from build123d import *

# Parameters (mm, degrees)
SKETCH1_R           = 2.7
BOSS_EXTRUDE1_DEPTH = 4


with BuildPart() as part:
    # Sketch1 → Boss-Extrude1 (new body)
    with BuildSketch(Plane(origin=(0, 0, 0), x_dir=(1, 0, 0), z_dir=(0, 1, 0))):
        with BuildLine():
            Line((13, 6.916598833), (13, -6.083401167))
            add(Edge.make_bspline(
                [(13, -6.083401167), (11.881455284, -6.181548449), (9.882372116, -6.337878454), (7.880965391, -6.456052029), (7, -6.5)],
                knots=[0, 0, 0, 0, 0.56, 1, 1, 1, 1], degree=3))
            add(Edge.make_bspline(
                [(7, -6.5), (6.834819068, -6.508242741), (6.666566964, -6.516342005), (5.350428343, -6.577459909), (3.178772662, -6.652062078), (1.020954011, -6.676072233), (-0.278468619, -6.676071849), (-1.578970751, -6.672116146), (-3.740363082, -6.635008847), (-5.632474881, -6.564362453), (-6.66657307, -6.516341675), (-6.834821325, -6.50824259), (-6.999999228, -6.5)],
                knots=[0, 0, 0, 0, 0.036447922, 0.036447922, 0.28, 0.500000307, 0.500000307, 0.56, 0.78, 0.963552693, 0.963552693, 1, 1, 1, 1], degree=3))
            add(Edge.make_bspline(
                [(-6.999999228, -6.5), (-8.121293995, -6.444062922), (-10.122381008, -6.320906395), (-12.121162985, -6.160515106), (-12.999999228, -6.083401167)],
                knots=[0, 0, 0, 0, 0.56, 1, 1, 1, 1], degree=3))
            Line((-12.999999228, -6.083401167), (-12.999999614, 6.916598833))
            add(Edge.make_bspline(
                [(-12.999999614, 6.916598833), (-11.002598721, 6.741335829), (-9.00219407, 6.599881753), (-7, 6.5)],
                knots=[1.5e-08, 1.5e-08, 1.5e-08, 1.5e-08, 0.230998109, 0.230998109, 0.230998109, 0.230998109], degree=3))
            Line((-7, 6.5), (7, 6.5))
            add(Edge.make_bspline(
                [(7, 6.5), (9.00219407, 6.599881753), (11.002598721, 6.741335829), (13, 6.916598833)],
                knots=[0.769001891, 0.769001891, 0.769001891, 0.769001891, 1, 1, 1, 1], degree=3))
        make_face()
        with Locations(Location((-7.5, 0, 0), (0, 0, 270))):
            Circle(SKETCH1_R, mode=Mode.SUBTRACT)
        with Locations(Location((7.5, 0, 0), (0, 0, 270))):
            Circle(SKETCH1_R, mode=Mode.SUBTRACT)
    extrude(amount=BOSS_EXTRUDE1_DEPTH)


solid = part.part
Read the model definition and answer for the solid it produces. Units are mm, in the model's axes. A direction names the side the tool comes from. Round coordinates to 2 decimals unless told otherwise and drop trailing zeros. Order: outer loops, then holes, each group sorted by start corner. A loop starts at its lowest first (then second) coordinate and runs counter-clockwise, first axis right, second up. Notation, with made-up numbers: (53.25, 89.5) - (62.25, 89.5) arc R14 ccw to (62.25, 100.5) - close; hole circle Ø2 at (-21.5, 76). An arc over 180 degrees is marked (long way). Use one line per item in the form item = value. Start each with the question number.
(1) The part is cut by section B-B (y = 1.55). Count the separate pieces of the cut face and the enclosed holes in it, then the cut area to 3 significant figures.
(2) For faces 1 (the face through (0, 2, -6.5)), 2 (the face through (0, 0, 0)), determine the directions among +Z, -Z, +X, -X, +Y, -Y from which every point of the face is accessible in a straight line to the end or side of a thin tool.
(3) Find the intervals of material crossed by line 1 along X through (y, z) = (1.3, 0); line 2 along X through (y, z) = (1.8, 0.75); line 3 along Z through (x, y) = (-8.5, 0.55), in increasing order. Write a range as from..to.
(4) The part is cut by section A-A (z = 0). Give the vertices of the cut face in (x, y), then the cut area to 3 significant figures.
(5) Determine the mould class of faces 3 (the face through (13, 2, -1)), 4 (the face through (5.105, 1.972, 1.246)), 5 (the face through (-9.895, 1.972, 1.246)), 6 (the face through (0, 4, 0)) for opening direction X: +X half, -X half, draft (parallel to the pull), parting line (faces both ways), or undercut.
(6) Flat-ended cylindrical pins translate along their axes: pin 1 Ø8 at (x, z) = (6.5, -1.5) entering from +Y; pin 2 Ø1.5 at (x, y) = (-0.5, 3) entering from -Z; pin 3 Ø5 at (x, z) = (-7.5, 0) entering from +Y. Find the tip coordinate at first contact, or state that the pin passes through.
Checked values:
q1.separate_pieces = 1
q1.enclosed_holes = 2
q1.area = 294 mm^2
q2.face_1 = -Z, +Y, -Y
q2.face_2 = +Z, -Z, +X, -X, -Y
q3.line_1 = -13..-10.2, -4.8..4.8, 10.2..13
q3.line_2 = -13..-10.09, -4.91..4.91, 10.09..13
q3.line_3 = -6.58..-2.51, 2.51..6.42
q4.outline = (-13, 0) - (-10.2, 0) - (-10.2, 4) - (-13, 4) - close; (-4.8, 0) - (4.8, 0) - (4.8, 4) - (-4.8, 4) - close; (10.2, 0) - (13, 0) - (13, 4) - (10.2, 4) - close
q4.area = 60.8 mm^2
q5.face_3 = +X half
q5.face_4 = undercut
q5.face_5 = undercut
q5.face_6 = draft
q6.pin_1 = 4
q6.pin_2 = -6.5
q6.pin_3 = through
